Check sheet for the modelled part. Datum: model origin and axes. Units: mm. Give positions to 0.01 mm unless a question says otherwise; leave off trailing zeros. Write each loop counter-clockwise with the first axis right and the second up, starting at its lowest first coordinate (ties: lowest second). Pieces come first, ordered by that corner, then holes. Notation, with made-up numbers: M 11,-2 L 20,-2 A32 ccw 20,25 Z; hole C 54.5,67 d6. An arc over 180 degrees is marked long. Write item = value, one per line. Start each with the question number.
1) Scan lines: L1, parallel to Y at x = 6.18, z = 1.2; L2, parallel to Y at x = 19, z = 1.5; L3, parallel to Y at x = 14, z = 1.4. Record each from-to range of solid material in increasing order.
2) Sectioned sample at B-B, the plane z = 0.9. Count the separate pieces of the cut face and the enclosed holes in it, then the cut area to 3 significant figures.
3) Sectioned sample at A-A, the plane y = 34. Record the cut outline in (x, z).
4) Draft check along X on faces 1 (the face through (35.5, 18, 1)), 2 (the face through (18, 19, 0)), 3 (the face through (2.03, 34.49, 0.79)). Enter one of: pulls with the +X half, pulls with the -X half, needs draft (parallel to the pull), parting line crosses it, or undercut.
from build123d import *

# Parameters (mm, degrees)
CYLINDER008_R     = 0.35
CYLINDER008_DEPTH = 1.6
CYLINDER009_R     = 0.35
CYLINDER009_DEPTH = 1.6
CYLINDER013_R     = 0.35
CYLINDER013_DEPTH = 1.6
CYLINDER018_R     = 0.35
CYLINDER018_DEPTH = 1.6
CYLINDER012_R     = 0.35
CYLINDER012_DEPTH = 1.6
CYLINDER015_R     = 0.35
CYLINDER015_DEPTH = 1.6
CYLINDER014_R     = 0.35
CYLINDER014_DEPTH = 1.6
CYLINDER016_R     = 0.35
CYLINDER016_DEPTH = 1.6
CYLINDER011_R     = 0.35
CYLINDER011_DEPTH = 1.6
CYLINDER010_R     = 0.35
CYLINDER010_DEPTH = 1.6
CYLINDER019_R     = 0.35
CYLINDER019_DEPTH = 1.6
CYLINDER020_R     = 0.35
CYLINDER020_DEPTH = 1.6
CYLINDER017_R     = 0.35
CYLINDER017_DEPTH = 1.6
CYLINDER004_R     = 0.35
CYLINDER004_DEPTH = 1.6
CYLINDER002_R     = 1.3
CYLINDER002_DEPTH = 1.6
CYLINDER001_R     = 1.3
CYLINDER001_DEPTH = 1.6
CYLINDER_R        = 1.3
CYLINDER_DEPTH    = 1.6
BOX_W             = 35.5
BOX_H             = 36.8
BOX_DEPTH         = 1.6


with BuildPart() as cylinder008:
    # Cylinder008 → Cylinder008 (new body)
    with BuildSketch(Plane(origin=(1.1, 12.7, 0), x_dir=(1, 0, 0), z_dir=(0, 0, 1))):
        Circle(CYLINDER008_R)
    extrude(amount=CYLINDER008_DEPTH)


with BuildPart() as cylinder009:
    # Cylinder009 → Cylinder009 (new body)
    with BuildSketch(Plane(origin=(8.72, 12.7, 0), x_dir=(1, 0, 0), z_dir=(0, 0, 1))):
        Circle(CYLINDER009_R)
    extrude(amount=CYLINDER009_DEPTH)


with BuildPart() as cylinder013:
    # Cylinder013 → Cylinder013 (new body)
    with BuildSketch(Plane(origin=(18.88, 12.7, 0), x_dir=(1, 0, 0), z_dir=(0, 0, 1))):
        Circle(CYLINDER013_R)
    extrude(amount=CYLINDER013_DEPTH)


with BuildPart() as cylinder018:
    # Cylinder018 → Cylinder018 (new body)
    with BuildSketch(Plane(origin=(34.12, 12.7, 0), x_dir=(1, 0, 0), z_dir=(0, 0, 1))):
        Circle(CYLINDER018_R)
    extrude(amount=CYLINDER018_DEPTH)


with BuildPart() as cylinder012:
    # Cylinder012 → Cylinder012 (new body)
    with BuildSketch(Plane(origin=(13.8, 12.7, 0), x_dir=(1, 0, 0), z_dir=(0, 0, 1))):
        Circle(CYLINDER012_R)
    extrude(amount=CYLINDER012_DEPTH)


with BuildPart() as cylinder015:
    # Cylinder015 → Cylinder015 (new body)
    with BuildSketch(Plane(origin=(21.42, 12.7, 0), x_dir=(1, 0, 0), z_dir=(0, 0, 1))):
        Circle(CYLINDER015_R)
    extrude(amount=CYLINDER015_DEPTH)


with BuildPart() as cylinder014:
    # Cylinder014 → Cylinder014 (new body)
    with BuildSketch(Plane(origin=(23.96, 12.7, 0), x_dir=(1, 0, 0), z_dir=(0, 0, 1))):
        Circle(CYLINDER014_R)
    extrude(amount=CYLINDER014_DEPTH)


with BuildPart() as cylinder016:
    # Cylinder016 → Cylinder016 (new body)
    with BuildSketch(Plane(origin=(16.34, 12.7, 0), x_dir=(1, 0, 0), z_dir=(0, 0, 1))):
        Circle(CYLINDER016_R)
    extrude(amount=CYLINDER016_DEPTH)


with BuildPart() as cylinder011:
    # Cylinder011 → Cylinder011 (new body)
    with BuildSketch(Plane(origin=(11.26, 12.7, 0), x_dir=(1, 0, 0), z_dir=(0, 0, 1))):
        Circle(CYLINDER011_R)
    extrude(amount=CYLINDER011_DEPTH)


with BuildPart() as cylinder010:
    # Cylinder010 → Cylinder010 (new body)
    with BuildSketch(Plane(origin=(6.18, 12.7, 0), x_dir=(1, 0, 0), z_dir=(0, 0, 1))):
        Circle(CYLINDER010_R)
    extrude(amount=CYLINDER010_DEPTH)


with BuildPart() as cylinder019:
    # Cylinder019 → Cylinder019 (new body)
    with BuildSketch(Plane(origin=(31.58, 12.7, 0), x_dir=(1, 0, 0), z_dir=(0, 0, 1))):
        Circle(CYLINDER019_R)
    extrude(amount=CYLINDER019_DEPTH)


with BuildPart() as cylinder020:
    # Cylinder020 → Cylinder020 (new body)
    with BuildSketch(Plane(origin=(26.5, 12.7, 0), x_dir=(1, 0, 0), z_dir=(0, 0, 1))):
        Circle(CYLINDER020_R)
    extrude(amount=CYLINDER020_DEPTH)


with BuildPart() as cylinder017:
    # Cylinder017 → Cylinder017 (new body)
    with BuildSketch(Plane(origin=(29.04, 12.7, 0), x_dir=(1, 0, 0), z_dir=(0, 0, 1))):
        Circle(CYLINDER017_R)
    extrude(amount=CYLINDER017_DEPTH)


with BuildPart() as cylinder004:
    # Cylinder004 → Cylinder004 (new body)
    with BuildSketch(Plane(origin=(3.64, 12.7, 0), x_dir=(1, 0, 0), z_dir=(0, 0, 1))):
        Circle(CYLINDER004_R)
    extrude(amount=CYLINDER004_DEPTH)


with BuildPart() as compound001:
    # Compound001 base: copy of Cylinder004
    add(cylinder004.part)

    # Compound001: union Cylinder008, Cylinder009, Cylinder013, Cylinder018, Cylinder012, Cylinder015, Cylinder014, Cylinder016, Cylinder011, Cylinder010, Cylinder019, Cylinder020, Cylinder017
    add(cylinder008.part)
    add(cylinder009.part)
    add(cylinder013.part)
    add(cylinder018.part)
    add(cylinder012.part)
    add(cylinder015.part)
    add(cylinder014.part)
    add(cylinder016.part)
    add(cylinder011.part)
    add(cylinder010.part)
    add(cylinder019.part)
    add(cylinder020.part)
    add(cylinder017.part)


with BuildPart() as compound001_1:
    # Compound001 placement: moved
    add(compound001.part.moved(Location((0, 15.24, 0))))


with BuildPart() as compound:
    # Compound base: copy of Cylinder004
    add(cylinder004.part)

    # Compound: union Cylinder008, Cylinder009, Cylinder013, Cylinder018, Cylinder012, Cylinder015, Cylinder014, Cylinder016, Cylinder011, Cylinder010, Cylinder019, Cylinder020, Cylinder017
    add(cylinder008.part)
    add(cylinder009.part)
    add(cylinder013.part)
    add(cylinder018.part)
    add(cylinder012.part)
    add(cylinder015.part)
    add(cylinder014.part)
    add(cylinder016.part)
    add(cylinder011.part)
    add(cylinder010.part)
    add(cylinder019.part)
    add(cylinder020.part)
    add(cylinder017.part)


with BuildPart() as cylinder002:
    # Cylinder002 → Cylinder002 (new body)
    with BuildSketch(Plane(origin=(32.2, 33.2, 0), x_dir=(1, 0, 0), z_dir=(0, 0, 1))):
        Circle(CYLINDER002_R)
    extrude(amount=CYLINDER002_DEPTH)


with BuildPart() as cylinder001:
    # Cylinder001 → Cylinder001 (new body)
    with BuildSketch(Plane(origin=(2.2, 33.2, 0), x_dir=(1, 0, 0), z_dir=(0, 0, 1))):
        Circle(CYLINDER001_R)
    extrude(amount=CYLINDER001_DEPTH)


with BuildPart() as cylinder:
    # Cylinder → Cylinder (new body)
    with BuildSketch(Plane(origin=(19.6, 2.9, 0), x_dir=(1, 0, 0), z_dir=(0, 0, 1))):
        Circle(CYLINDER_R)
    extrude(amount=CYLINDER_DEPTH)


with BuildPart() as main_board:
    # Box → Box (new body)
    with BuildSketch(Plane.XY):
        with Locations((17.75, 18.4)):
            Rectangle(BOX_W, BOX_H)
    extrude(amount=BOX_DEPTH)

    # Cut: cut Cylinder
    add(cylinder.part, mode=Mode.SUBTRACT)

    # Cut001: cut Cylinder001
    add(cylinder001.part, mode=Mode.SUBTRACT)

    # Cut002: cut Cylinder002
    add(cylinder002.part, mode=Mode.SUBTRACT)

    # Cut004: cut Compound
    add(compound.part, mode=Mode.SUBTRACT)

    # Cut005: cut Compound001
    add(compound001_1.part, mode=Mode.SUBTRACT)


solid = main_board.part
Data:
q1.L1 = 0 to 12.35, 13.05 to 27.59, 28.29 to 36.8
q1.L2 = 0 to 1.75, 4.05 to 12.37, 13.03 to 27.61, 28.27 to 36.8
q1.L3 = 0 to 12.41, 12.99 to 27.65, 28.23 to 36.8
q2.separate_pieces = 1
q2.enclosed_holes = 31
q2.area = 1,280 mm2
q3.outline = M 0,0 L 1.18,0 L 1.18,1.6 L 0,1.6 Z; M 3.22,0 L 31.18,0 L 31.18,1.6 L 3.22,1.6 Z; M 33.22,0 L 35.5,0 L 35.5,1.6 L 33.22,1.6 Z
q4.face_1 = pulls with the +X half
q4.face_2 = needs draft
q4.face_3 = undercut
